Model file for the job. Use its own axes, mm. Round coordinates to 2 decimals unless told otherwise and drop trailing zeros. Order: outer loops, then holes, each group sorted by start corner. A loop starts at its lowest first (then second) coordinate and runs counter-clockwise, first axis right, second up. Notation, with made-up numbers: (69, 2) - (116, 2) arc R14 cw to (116, 6) - close; hole circle Ø3 at (84.25, 2.25). An arc over 180 degrees is marked (long way). Write item = value, one per line.
```python
from build123d import *

# Parameters (mm, degrees)
SKETCH1_W           = 76
SKETCH1_H           = 76
SKETCH1_R           = 3
BOSS_EXTRUDE1_DEPTH = 10


with BuildPart() as part:
    # Sketch1 → Boss-Extrude1 (new body)
    with BuildSketch(Plane(origin=(0, 0, 0), x_dir=(1, 0, 0), z_dir=(0, 1, 0))):
        with Locations((-159.8596663, 81.710219679)):
            Rectangle(SKETCH1_W, SKETCH1_H)
        with Locations(Location((-159.8596663, 81.710219679, 0), (0, 0, 270))):
            Circle(SKETCH1_R, mode=Mode.SUBTRACT)
        with Locations(Location((-134.769453056, 81.710219679, 0), (0, 0, 270))):
            Circle(SKETCH1_R, mode=Mode.SUBTRACT)
        with Locations(Location((-184.949879544, 81.710219679, 0), (0, 0, 90))):
            Circle(SKETCH1_R, mode=Mode.SUBTRACT)
        with Locations(Location((-184.949879544, 106.710219679, 0), (0, 0, 90))):
            Circle(SKETCH1_R, mode=Mode.SUBTRACT)
        with Locations(Location((-159.8596663, 106.710219679, 0), (0, 0, 270))):
            Circle(SKETCH1_R, mode=Mode.SUBTRACT)
        with Locations(Location((-134.769453056, 106.710219679, 0), (0, 0, 270))):
            Circle(SKETCH1_R, mode=Mode.SUBTRACT)
        with Locations(Location((-134.769453056, 56.710219679, 0), (0, 0, 90))):
            Circle(SKETCH1_R, mode=Mode.SUBTRACT)
        with Locations(Location((-159.8596663, 56.710219679, 0), (0, 0, 90))):
            Circle(SKETCH1_R, mode=Mode.SUBTRACT)
        with Locations(Location((-184.949879544, 56.710219679, 0), (0, 0, 270))):
            Circle(SKETCH1_R, mode=Mode.SUBTRACT)
    extrude(amount=BOSS_EXTRUDE1_DEPTH)


solid = part.part
```
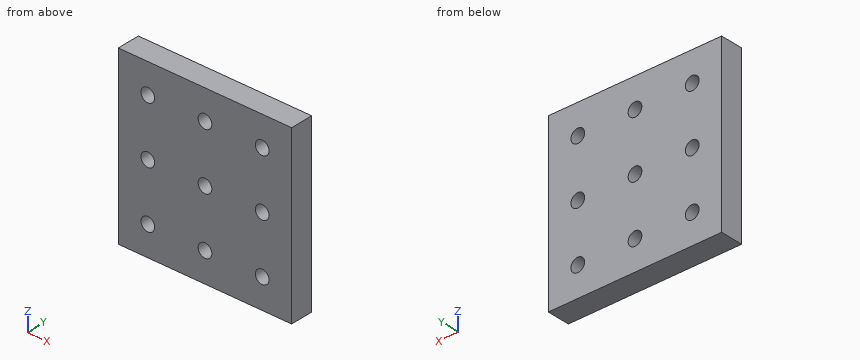
1) Cut at C-C (y = 6.5). Give the number of separate pieces and of enclosed holes in the cut face, and give its area (3 significant figures).
Conclusion:
separate_pieces = 1
enclosed_holes = 9
area = 5,520 mm^2
2) Cut at B-B (z = -83). Write the cut outline in (x, y), and give its area (3 significant figures).
Conclusion:
outline = (-197.86, 0) - (-187.66, 0) - (-187.66, 10) - (-197.86, 10) - close; (-182.24, 0) - (-162.57, 0) - (-162.57, 10) - (-182.24, 10) - close; (-157.15, 0) - (-137.48, 0) - (-137.48, 10) - (-157.15, 10) - close; (-132.06, 0) - (-121.86, 0) - (-121.86, 10) - (-132.06, 10) - close
area = 597 mm^2
3) Cut at A-A (x = -183.5). Write the cut outline in (y, z).
Conclusion:
outline = (0, -119.71) - (10, -119.71) - (10, -109.34) - (0, -109.34) - close; (0, -104.08) - (10, -104.08) - (10, -84.34) - (0, -84.34) - close; (0, -79.08) - (10, -79.08) - (10, -59.34) - (0, -59.34) - close; (0, -54.08) - (10, -54.08) - (10, -43.71) - (0, -43.71) - close
4) Wall check: line 1 along X through (y, z) = (4.5, -54.5); line 2 along X through (y, z) = (1.75, -83); line 3 along Z through (x, y) = (-158, 9.25). Give the ranges that are in metal, low to high.
Conclusion:
line_1 = -197.86 to -186.98, -182.92 to -161.89, -157.83 to -136.8, -132.74 to -121.86
line_2 = -197.86 to -187.66, -182.24 to -162.57, -157.15 to -137.48, -132.06 to -121.86
line_3 = -119.71 to -109.06, -104.36 to -84.06, -79.36 to -59.06, -54.36 to -43.71
5) Flat gauge pins, fed straight in: pin 1 Ø9.5 at (x, z) = (-159.86, -81.71) entering from +Y; pin 2 Ø5.5 at (x, z) = (-184.95, -106.71) entering from -Y. Where does each tip first touch, or does it go through?
Conclusion:
pin_1 = 10
pin_2 = through
